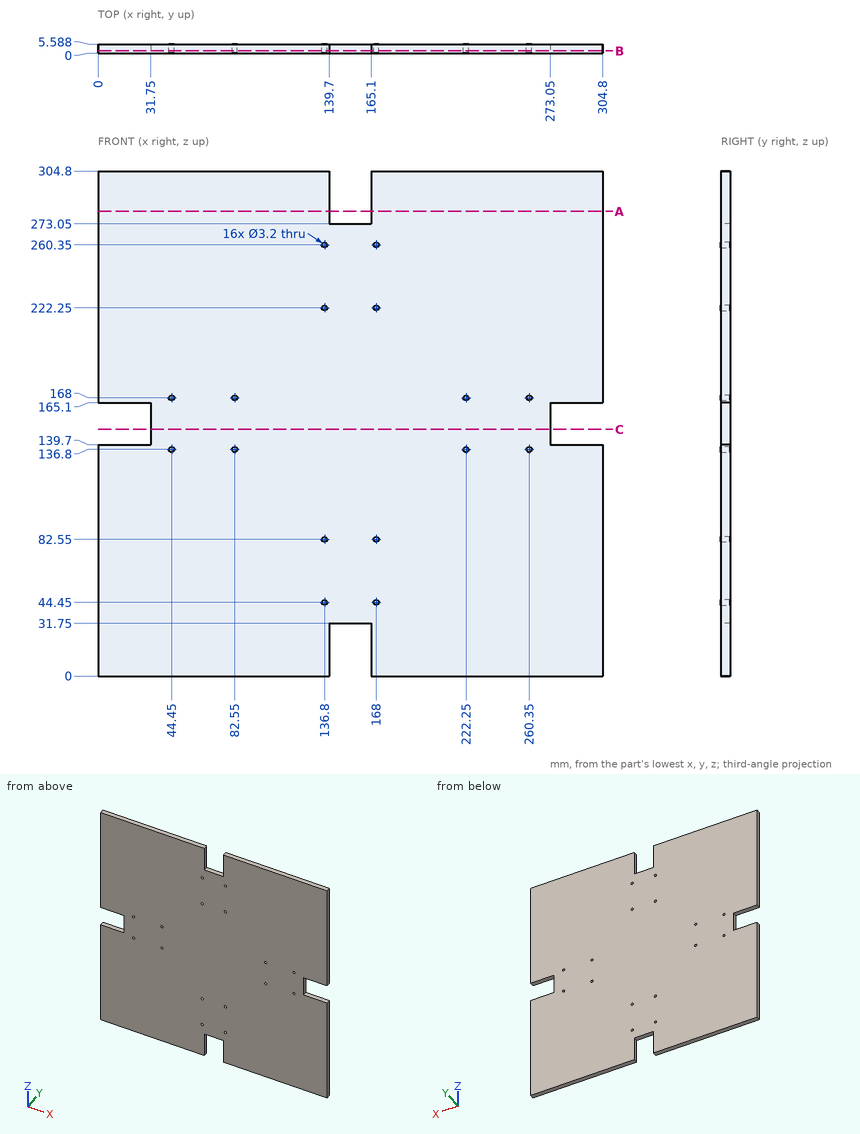
Check sheet for the drawn part. Datum: minimum x, y, z corner. Units: mm. Give positions to 0.01 mm unless a question says otherwise; leave off trailing zeros. Loops run counter-clockwise (first coordinate to the right, second up) from the corner with the lowest first, then second, coordinate; pieces in that order, holes last. Notation, with made-up numbers: M 85,31.5 L 92,31.5 A20 cw 92,48.5 Z; hole C -34,40 d10. An arc over 180 degrees is marked long. Answer as CSV lines item,"result".
Item 1: Scan lines: L1, parallel to X at y = 3.1, z = 168; L2, parallel to X at y = 4.15, z = 44.45. Record each from-to range of solid material in increasing order.
Reply:
L1,"0 to 42.85, 46.05 to 80.95, 84.15 to 220.65, 223.85 to 258.75, 261.95 to 304.8"
L2,"0 to 135.2, 138.4 to 166.4, 169.6 to 304.8"
Item 2: Sectioned sample at C-C, the plane z = 149. Enter the section's corners in (x, y).
Reply:
outline,"M 31.75,0 L 273.05,0 L 273.05,5.59 L 31.75,5.59 Z"
Item 3: Sectioned sample at B-B, the plane y = 1.4. State how many separate pieces and enclosed holes the cut face has, then the cut area to 3 significant figures.
Reply:
separate pieces,"1"
enclosed holes,"16"
area,"89,500 mm^2"
Item 4: Sectioned sample at A-A, the plane z = 280.5. Enter the section's corners in (x, y), then the cut area to 3 significant figures.
Reply:
outline,"M 0,0 L 139.7,0 L 139.7,5.59 L 0,5.59 Z; M 165.1,0 L 304.8,0 L 304.8,5.59 L 165.1,5.59 Z"
area,"1,560 mm^2"
Item 5: Depth check by flat-ended pin: pin 1 Ø1.7 at (x, y) = (11, 2) entering from -Z; pin 2 Ø3 at (x, z) = (136.8, 222.25) entering from -Y; pin 3 Ø3 at (y, z) = (3, 143.5) entering from +X; pin 4 Ø2 at (x, y) = (141, 3) entering from +Z. Enter the tip coordinate at first touch or a pass-through.
Reply:
pin 1,"z = 0"
pin 2,"through"
pin 3,"x = 273.05"
pin 4,"z = 273.05"
